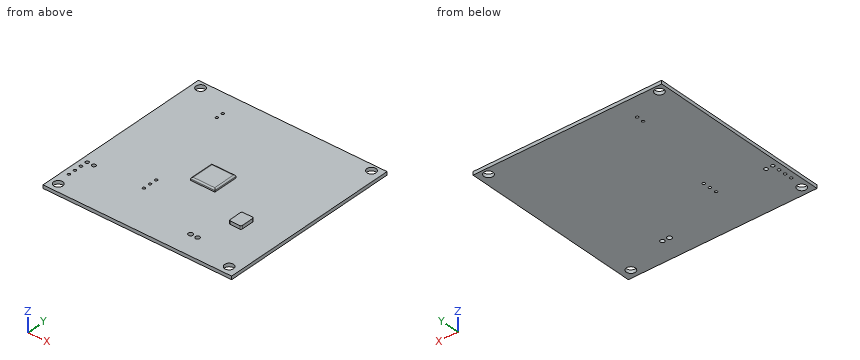
from build123d import *

# Parameters (mm, degrees)
ESQUISSE1_W        = 68.1
ESQUISSE1_H        = 66.15
ESQUISSE1_R        = 1.625
ESQUISSE1_R_2      = 0.5199497
ESQUISSE1_R_3      = 0.496597476
ESQUISSE1_R_4      = 0.485049202
ESQUISSE1_R_5      = 0.608998307
ESQUISSE1_R_6      = 0.677903493
ESQUISSE1_R_7      = 0.838572367
ESQUISSE1_R_8      = 0.778774178
ESQUISSE1_R_9      = 0.487785526
ESQUISSE1_R_10     = 0.479472078
ESQUISSE1_R_11     = 0.483052504
ESQUISSE1_R_12     = 0.489527541
ESQUISSE1_R_13     = 0.470271612
BOSS_EXTRU_1_DEPTH = 1.2
ESQUISSE3_W        = 8.757871462
ESQUISSE3_H        = 8.976039079
BOSS_EXTRU_2_DEPTH = 1
CONG_1_R           = 0.5
ESQUISSE4_W        = 4.395615229
ESQUISSE4_H        = 5.378660169
BOSS_EXTRU_3_DEPTH = 1.2
CONG_2_R           = 0.5


with BuildPart() as part:
    # Esquisse1 → Boss.-Extru.1 (new body)
    with BuildSketch(Plane.XY):
        with Locations((52.364343219, 246.888419198)):
            Rectangle(ESQUISSE1_W, ESQUISSE1_H)
        with Locations((21.20400612, 216.902097721)):
            Circle(ESQUISSE1_R, mode=Mode.SUBTRACT)
        with Locations((82.892966431, 216.902097721)):
            Circle(ESQUISSE1_R, mode=Mode.SUBTRACT)
        with Locations((21.20400612, 277.517138812)):
            Circle(ESQUISSE1_R, mode=Mode.SUBTRACT)
        with Locations((82.892966431, 277.517138812)):
            Circle(ESQUISSE1_R, mode=Mode.SUBTRACT)
        with Locations((20.460946771, 227.424751553)):
            Circle(ESQUISSE1_R_2, mode=Mode.SUBTRACT)
        with Locations((20.460946771, 224.857942008)):
            Circle(ESQUISSE1_R_3, mode=Mode.SUBTRACT)
        with Locations((20.428852881, 222.304104047)):
            Circle(ESQUISSE1_R_4, mode=Mode.SUBTRACT)
        with Locations((20.539364867, 230.017790559)):
            Circle(ESQUISSE1_R_5, mode=Mode.SUBTRACT)
        with Locations((22.937900475, 230.017790559)):
            Circle(ESQUISSE1_R_6, mode=Mode.SUBTRACT)
        with Locations((64.715000433, 221.952763309)):
            Circle(ESQUISSE1_R_7, mode=Mode.SUBTRACT)
        with Locations((67.21953945, 221.952763309)):
            Circle(ESQUISSE1_R_8, mode=Mode.SUBTRACT)
        with Locations((40.53207734, 235.781211634)):
            Circle(ESQUISSE1_R_9, mode=Mode.SUBTRACT)
        with Locations((40.53207734, 233.196854691)):
            Circle(ESQUISSE1_R_10, mode=Mode.SUBTRACT)
        with Locations((40.53207734, 230.561657941)):
            Circle(ESQUISSE1_R_11, mode=Mode.SUBTRACT)
        with Locations((33.847033777, 272.050619819)):
            Circle(ESQUISSE1_R_12, mode=Mode.SUBTRACT)
        with Locations((33.847033777, 269.501928251)):
            Circle(ESQUISSE1_R_13, mode=Mode.SUBTRACT)
    extrude(amount=-BOSS_EXTRU_1_DEPTH)

    # Esquisse3 → Boss.-Extru.2 (add)
    with BuildSketch(Plane.XY):
        with Locations((52.308376614, 246.236021207)):
            Rectangle(ESQUISSE3_W, ESQUISSE3_H)
    extrude(amount=BOSS_EXTRU_2_DEPTH)

    # Congé1
    cong_1_edges = [part.edges().sort_by_distance(p)[0] for p in [
        (47.929440883, 246.236021207, 1),
        (52.308376614, 241.748001667, 1),
        (56.687312345, 246.236021207, 1),
        (52.308376614, 250.724040746, 1),
    ]]
    fillet(cong_1_edges, radius=CONG_1_R)

    # Esquisse4 → Boss.-Extru.3 (add)
    with BuildSketch(Plane.XY):
        with Locations((71.755113955, 235.261974176)):
            Rectangle(ESQUISSE4_W, ESQUISSE4_H)
    extrude(amount=BOSS_EXTRU_3_DEPTH)

    # Congé2
    cong_2_edges = [part.edges().sort_by_distance(p)[0] for p in [
        (69.55730634, 237.95130426, 0.6),
        (69.55730634, 232.572644091, 0.6),
        (73.952921569, 232.572644091, 0.6),
        (73.952921569, 237.95130426, 0.6),
    ]]
    fillet(cong_2_edges, radius=CONG_2_R)


solid = part.part
Check sheet for the modelled part. Datum: model origin and axes. Units: mm. Give positions to 0.01 mm unless a question says otherwise; leave off trailing zeros. Loops run counter-clockwise (first coordinate to the right, second up) from the corner with the lowest first, then second, coordinate; pieces in that order, holes last. Notation, with made-up numbers: M -35,75 L 12,75 A17 cw 12,104 Z; hole C 12,35 d5. An arc over 180 degrees is marked long. Use a Markdown table: item, result. Add a question column.
Q1. Sectioned sample at C-C, the plane y = 258.5. Record the cut outline in (x, z).
Q2. Sectioned sample at B-B, the plane x = 39. Record the cut outline in (y, z).
Q3. Sectioned sample at A-A, the plane y = 246.5. Record the cut outline in (x, z), then the cut area to 3 significant figures.
Q4. Go/stop test with flat-tipped pins: pin 1 (0.6 mm diameter, centred on x = 72, z = 0.5, fed in from -Y); pin 2 (6 mm diameter, centred on x = 51.5, y = 247, fed in from +Z); pin 3 (3.5 mm diameter, centred on x = 82.89, y = 277.52, fed in from +Z). Record where each tip stops, or that it passes through.
Q5. Scan lines: line 1 along Y through (x, z) = (23, -1.05); line 2 along Y through (x, z) = (81.5, -0.05); line 3 along Z through (x, y) = (55, 260). Record each from-to range of solid material in increasing order. Write a range as [from, to].
Verdict:
| question | item | result |
|---|---|---|
| 1 | outline | M 18.31,-1.2 L 86.41,-1.2 L 86.41,0 L 18.31,0 Z |
| 2 | outline | M 213.81,-1.2 L 279.96,-1.2 L 279.96,0 L 213.81,0 Z |
| 3 | outline | M 18.31,-1.2 L 86.41,-1.2 L 86.41,0 L 56.69,0 L 56.69,0.5 A0.5 ccw 56.19,1 L 48.43,1 A0.5 ccw 47.93,0.5 L 47.93,0 L 18.31,0 Z |
| 3 | area | 90.4 mm^2 |
| 4 | pin 1 | y = 232.57 |
| 4 | pin 2 | z = 1 |
| 4 | pin 3 | z = 0 |
| 5 | line 1 | [213.81, 229.34], [230.69, 279.96] |
| 5 | line 2 | [213.81, 216.07], [217.74, 276.68], [278.35, 279.96] |
| 5 | line 3 | [-1.2, 0] |
